```python
from build123d import *

# Parameters (mm, degrees)
F0_W     = 152.4
F0_H     = 304.8
F1_DEPTH = 76.2
F2_R     = 5.08
F3_T     = 5.08
F4_W     = 127
F4_H     = 254
F5_DEPTH = 25.4
F6_W     = 40
F6_H     = 40
F7_DEPTH = 5.08


# Not quite as in the source:
# - a shell that OpenCascade refuses in one call is made with other operations: the cavity is built on its own and cut out


with BuildPart() as f1:
    # F0 (on Front) → F1 (new body, symmetric)
    with BuildSketch(Plane.XZ):
        Rectangle(F0_W, F0_H)
    extrude(amount=F1_DEPTH, both=True)

    # F2
    f2_edges = [f1.edges().sort_by_distance(p)[0] for p in [
        (0, -76.2, 152.4),
        (76.2, 0, 152.4),
        (76.2, -76.2, 0),
        (76.2, 76.2, 0),
        (0, 76.2, 152.4),
        (-76.2, 0, 152.4),
        (-76.2, -76.2, 0),
        (-76.2, 76.2, 0),
    ]]
    fillet(f2_edges, radius=F2_R)

    # F3: shell of thickness 5.08, made by hand


with BuildPart() as f3_core1:
    # F3_t2: copy of F1
    add(f1.part)

    # the walls: a layer under each face that stays
    f3_faces = [f3_core1.faces().sort_by_distance(p)[0] for p in [
        (0, 0, -152.4),
        (0, 76.2, -2.54),
        (-76.2, 0, -2.54),
        (76.2, 0, -2.54),
        (0, -76.2, -2.54),
        (0, 0, 152.4),
    ]]
    thicken(f3_faces, amount=-F3_T, mode=Mode.SUBTRACT)


with BuildPart() as f1_1:
    add(f1.part)

    # what is left inside the walls is the cavity
    f3_cavity = [f3_core1.part.solids().sort_by_distance(p)[0] for p in [
        (-71.0692, 23.706667, 0),
    ]]
    add(f3_cavity, mode=Mode.SUBTRACT)

    # F4 (on face) → F5 (cut)
    with BuildSketch(Plane.XZ.offset(76.2)):
        Rectangle(F4_W, F4_H)
    extrude(amount=-F5_DEPTH, mode=Mode.SUBTRACT)

    # F6 (on face) → F7 (cut)
    with BuildSketch(Plane.XY.offset(152.4)):
        Rectangle(F6_W, F6_H)
    extrude(amount=-F7_DEPTH, mode=Mode.SUBTRACT)


solid = f1_1.part
```
Verification items for the finished model (mm, model axes). A direction names the side the tool comes from. Coordinates: 2 decimals unless noted, no trailing zeros. Write each loop counter-clockwise with the first axis right and the second up, starting at its lowest first coordinate (ties: lowest second). Pieces come first, ordered by that corner, then holes. Notation, with made-up numbers: (79, 65.25) - (116, 65.25) arc R19 ccw to (116, 79.25) - close; hole circle Ø9 at (58, -15.5). An arc over 180 degrees is marked (long way). One line per question, with ' | ' between items. Start each with the question number.
1. Gauge pin test, flat ends, axial feed: P1, Ø5.5, axis at y = 7.5, z = 149, coming from the +X side; P2, Ø1.5, axis at y = 7, z = 151, coming from the -X side; P3, Ø1.5, axis at y = -73.5, z = -52, coming from the +X side; P4, Ø4, axis at x = 9.5, y = -73.5, coming from the +Z side. Record the tip position at first contact, or that the pin passes through.
2. Draft check along X on faces 1 (the flat face through (-64, -71.12, -10)), 2 (the flat face through (-76.2, -1, -5)), 3 (the flat face through (31, -1, 152.4)). Enter one of: released by +X, released by -X, zero draft, split by the parting line, or undercut.
3. Access from +Z, -Z, +X, -X, +Y, -Y to the whole of each face (thin tool, end or side, straight path). Record for faces 4 (the flat face through (-1, -1, -152.4)), 5 (the flat face through (31, -1, 147.32)).
4. Material ranges on line 1 along X through (y, z) = (60.5, -69); line 2 along Z through (x, y) = (66.5, 38.5), recorded low to high.
5. Section check D-D (x = 27.5). Enter the section's corners in (y, z), plus the area to 3 significant figures.
6. Section check A-A (x = -16.5). Enter the section's corners in (y, z).
7. Section check C-C (z = 7). Enter the section's corners in (x, y), plus the area to 3 significant figures.
8. Section check B-B (y = 60.5). Enter the section's corners in (x, z), plus the area to 3 significant figures.
Computed values:
1) P1: x = 76.2 | P2: x = -75.27 | P3: x = 75.93 | P4: z = 152.39
2) face 1: undercut | face 2: released by -X | face 3: zero draft
3) face 4: -Z, +X, -X, +Y, -Y | face 5: none
4) line 1: -76.2 to -71.12, 71.12 to 76.2 | line 2: -152.4 to -147.32, 147.32 to 152.4
5) outline: (-76.2, -152.4) - (76.2, -152.4) - (76.2, 147.32) arc R5.08 ccw to (71.12, 152.4) - (-71.12, 152.4) arc R5.08 ccw to (-76.2, 147.32) - (-76.2, 127) - (-71.12, 127) - (-71.12, 147.32) - (71.12, 147.32) - (71.12, -147.32) - (-71.12, -147.32) - (-71.12, -127) - (-76.2, -127) - close | area: 3,240 mm²
6) outline: (-76.2, -152.4) - (76.2, -152.4) - (76.2, 147.32) arc R5.08 ccw to (71.12, 152.4) - (20, 152.4) - (20, 147.32) - (71.12, 147.32) - (71.12, -147.32) - (-71.12, -147.32) - (-71.12, -127) - (-76.2, -127) - close; (-76.2, 127) - (-71.12, 127) - (-71.12, 147.32) - (-20, 147.32) - (-20, 152.4) - (-71.12, 152.4) arc R5.08 ccw to (-76.2, 147.32) - close
7) outline: (-76.2, -71.12) arc R5.08 ccw to (-71.12, -76.2) - (-63.5, -76.2) - (-63.5, -71.12) - (-71.12, -71.12) - (-71.12, 71.12) - (71.12, 71.12) - (71.12, -71.12) - (63.5, -71.12) - (63.5, -76.2) - (71.12, -76.2) arc R5.08 ccw to (76.2, -71.12) - (76.2, 71.12) arc R5.08 ccw to (71.12, 76.2) - (-71.12, 76.2) arc R5.08 ccw to (-76.2, 71.12) - close | area: 2,330 mm²
8) outline: (-76.2, -152.4) - (76.2, -152.4) - (76.2, 147.32) arc R5.08 ccw to (71.12, 152.4) - (-71.12, 152.4) arc R5.08 ccw to (-76.2, 147.32) - close; hole (-71.12, -147.32) - (71.12, -147.32) - (71.12, 147.32) - (-71.12, 147.32) - close | area: 4,530 mm²
